from build123d import *

# Parameters (mm, degrees)
SKETCH1_R           = 75
BOSS_EXTRUDE1_DEPTH = 3
SKETCH2_W           = 10
SKETCH2_H           = 40
CUT_EXTRUDE1_DEPTH  = 6.35
SKETCH8_R           = 1.7145
CUT_EXTRUDE7_DEPTH  = 4
SKETCH9_W           = 30
SKETCH9_H           = 15
CUT_EXTRUDE8_DEPTH  = 4
FILLET1_R           = 5
SKETCH10_R          = 1.7145
CUT_EXTRUDE9_DEPTH  = 10


with BuildPart() as part:
    # Sketch1 → Boss-Extrude1 (new body)
    with BuildSketch(Plane(origin=(0, 0, 0), x_dir=(1, 0, 0), z_dir=(0, 1, 0))):
        Circle(SKETCH1_R)
    extrude(amount=BOSS_EXTRUDE1_DEPTH)

    # Sketch2 → Cut-Extrude1 (cut)
    with BuildSketch(Plane(origin=(0, 3, 0), x_dir=(1, 0, 0), z_dir=(0, 1, 0))):
        with Locations((-61, 0)):
            Rectangle(SKETCH2_W, SKETCH2_H)
        with Locations((61, 0)):
            Rectangle(SKETCH2_W, SKETCH2_H)
    extrude(amount=-CUT_EXTRUDE1_DEPTH, mode=Mode.SUBTRACT)

    # Sketch8 → Cut-Extrude7 (cut, through all)
    with BuildSketch(Plane(origin=(0, 3, 0), x_dir=(1, 0, 0), z_dir=(0, 1, 0))):
        with Locations((-45, 45)):
            Circle(SKETCH8_R)
        with Locations((45, 45)):
            Circle(SKETCH8_R)
        with Locations((45, -45)):
            Circle(SKETCH8_R)
        with Locations((-45, -45)):
            Circle(SKETCH8_R)
    extrude(amount=-CUT_EXTRUDE7_DEPTH, mode=Mode.SUBTRACT)

    # Sketch9 → Cut-Extrude8 (cut, through all)
    with BuildSketch(Plane(origin=(0, 3, 0), x_dir=(1, 0, 0), z_dir=(0, 1, 0))):
        Rectangle(SKETCH9_W, SKETCH9_H)
    extrude(amount=-CUT_EXTRUDE8_DEPTH, mode=Mode.SUBTRACT)

    # Fillet1
    fillet1_edges = [part.edges().sort_by_distance(p)[0] for p in [
        (15, 1.5, -7.5),
        (15, 1.5, 7.5),
        (-15, 1.5, 7.5),
        (-15, 1.5, -7.5),
    ]]
    fillet(fillet1_edges, radius=FILLET1_R)

    # Sketch10 → Cut-Extrude9 (cut)
    with BuildSketch(Plane(origin=(0, 3, 0), x_dir=(1, 0, 0), z_dir=(0, 1, 0))):
        with Locations((34.29, 59.09)):
            Circle(SKETCH10_R)
        with Locations((34.29, 15.91)):
            Circle(SKETCH10_R)
        with Locations((-34.29, 15.91)):
            Circle(SKETCH10_R)
        with Locations((-34.29, 59.09)):
            Circle(SKETCH10_R)
        with Locations((-34.29, -15.91)):
            Circle(SKETCH10_R)
        with Locations((-34.29, -59.09)):
            Circle(SKETCH10_R)
        with Locations((34.29, -59.09)):
            Circle(SKETCH10_R)
        with Locations((34.29, -15.91)):
            Circle(SKETCH10_R)
    extrude(amount=-CUT_EXTRUDE9_DEPTH, mode=Mode.SUBTRACT)


solid = part.part
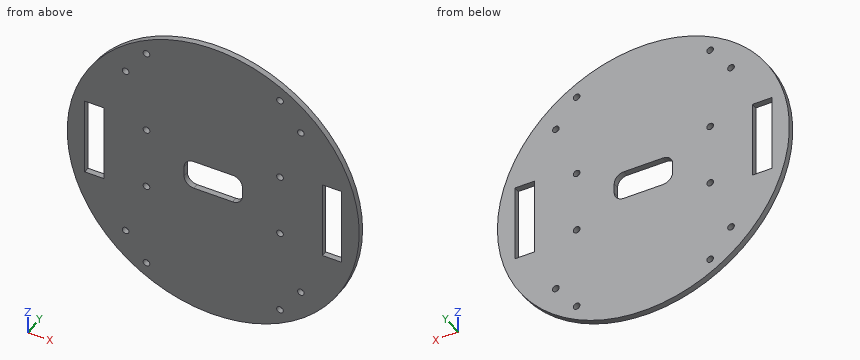
Can you work these out from the model? Positions are in its coordinate system, mm. Give positions to 0.01 mm unless a question says otherwise; leave off trailing zeros. Write each loop counter-clockwise with the first axis right and the second up, starting at its lowest first coordinate (ties: lowest second). Pieces come first, ordered by that corner, then holes. Notation, with made-up numbers: (12.5, -19) -> (35.5, -19) arc R16 ccw to (35.5, 5) -> close; hole circle Ø10 at (72.25, 32.5). An arc over 180 degrees is marked (long way). Answer as a JSON object with one key per item and string values. Group by question number.
Item 1: Suppose I cut it at D-D (x = 0). Please give me the cut outline in (y, z).
Item 2: Please list where these lines run through material, in increasing order: line 1 (Z direction, x = -34.29, y = 2.3); line 2 (X direction, y = 0.4, z = 11); line 3 (Z direction, x = 45, y = 1.1). Write a range as [from, to].
Item 3: Suppose I cut it at A-A (z = 0). Please give me the cut outline in (x, y), plus the area to 3 significant figures.
Item 4: I'm going to push flat-ended pins straight in: P1, Ø0.9, axis at x = 5, y = 2, coming from the -Z side; P2, Ø0.9, axis at y = 2, z = -5.5, coming from the +X side; P3, Ø2, axis at x = -34.29, z = 15.91, coming from the -Y side. Where does each tip first touch, or does it pass through?
Item 5: Suppose I cut it at B-B (z = 45). Please give me the cut outline in (x, y).
Item 6: Suppose I cut it at C-C (y = 1.15). State how many separate pieces and enclosed holes the cut face has, plus the area to 3 significant figures.
Findings:
{
 "1": {"outline": "(0, -75) -> (3, -75) -> (3, -7.5) -> (0, -7.5) -> close; (0, 7.5) -> (3, 7.5) -> (3, 75) -> (0, 75) -> close"},
 "2": {"line 1": "z = [-66.7, -60.8], [-57.38, -17.62], [-14.2, 14.2], [17.62, 57.38], [60.8, 66.7]", "line 2": "x = [-74.19, -66], [-56, 56], [66, 74.19]", "line 3": "z = [-60, -46.71], [-43.29, 43.29], [46.71, 60]"},
 "3": {"outline": "(-75, 0) -> (-66, 0) -> (-66, 3) -> (-75, 3) -> close; (-56, 0) -> (-15, 0) -> (-15, 3) -> (-56, 3) -> close; (15, 0) -> (56, 0) -> (56, 3) -> (15, 3) -> close; (66, 0) -> (75, 0) -> (75, 3) -> (66, 3) -> close", "area": "300 mm²"},
 "4": {"P1": "stops at z = -74.86", "P2": "stops at x = 74.83", "P3": "passes through"},
 "5": {"outline": "(-60, 0) -> (-46.71, 0) -> (-46.71, 3) -> (-60, 3) -> close; (-43.29, 0) -> (43.29, 0) -> (43.29, 3) -> (-43.29, 3) -> close; (46.71, 0) -> (60, 0) -> (60, 3) -> (46.71, 3) -> close"},
 "6": {"separate pieces": "1", "enclosed holes": "15", "area": "16,300 mm²"}
}
